```python
from build123d import *

# Parameters (mm, degrees)
BOSS_EXTRUDE1_DEPTH = 35.56
SKETCH2_W           = 2.54
SKETCH2_H           = 5.08
CUT_EXTRUDE1_DEPTH  = 10.16
SKETCH3_W           = 2.54
SKETCH3_H           = 5.08
CUT_EXTRUDE2_DEPTH  = 10.16
CHAMFER1_SIZE       = 0.508
FILLET1_R           = 0.635


with BuildPart() as part:
    # Sketch1 → Boss-Extrude1 (new body)
    with BuildSketch(Plane.XY):
        Polygon((-19.05, -0.3175), (-19.05, 0.3175), (-1.27, 0.3175), (-1.27, 5.3975), (1.27, 5.3975), (1.27, 0.3175), (19.05, 0.3175), (19.05, -0.3175), (1.27, -0.3175), (1.27, -0.635), (19.05, -0.635), (19.05, -1.27), (-19.05, -1.27), (-19.05, -0.635), (-1.27, -0.635), (-1.27, -0.3175), align=None)
    extrude(amount=-BOSS_EXTRUDE1_DEPTH)

    # Sketch2 → Cut-Extrude1 (cut)
    with BuildSketch(Plane.XY):
        with Locations((0, 2.8575)):
            Rectangle(SKETCH2_W, SKETCH2_H)
    extrude(amount=-CUT_EXTRUDE1_DEPTH, mode=Mode.SUBTRACT)

    # Sketch3 → Cut-Extrude2 (cut)
    with BuildSketch(Plane(origin=(0, 0, -35.56), x_dir=(-1, 0, 0), z_dir=(0, 0, -1))):
        with Locations((0, 2.8575)):
            Rectangle(SKETCH3_W, SKETCH3_H)
    extrude(amount=-CUT_EXTRUDE2_DEPTH, mode=Mode.SUBTRACT)

    # Chamfer1
    chamfer1_edges = [part.edges().sort_by_distance(p)[0] for p in [
        (0, 5.3975, -10.16),
        (1.27, 5.3975, -17.78),
        (-1.27, 5.3975, -17.78),
        (0, 5.3975, -25.4),
    ]]
    chamfer(chamfer1_edges, length=CHAMFER1_SIZE)

    # Fillet1
    fillet1_edges = [part.edges().sort_by_distance(p)[0] for p in [
        (1.27, 4.8895, -17.78),
        (0, 5.3975, -24.892),
        (-0.762, 5.3975, -17.78),
        (0, 5.3975, -10.668),
        (0.762, 5.3975, -17.78),
        (0, 4.8895, -10.16),
        (-1.27, 4.8895, -17.78),
        (0, 4.8895, -25.4),
    ]]
    fillet(fillet1_edges, radius=FILLET1_R)


solid = part.part
```
Check sheet for the modelled part. Datum: model origin and axes. Units: mm. A direction names the side the tool comes from. Coordinates: 2 decimals unless noted, no trailing zeros. Loops run counter-clockwise (first coordinate to the right, second up) from the corner with the lowest first, then second, coordinate; pieces in that order, holes last.
1) Material ranges on probe 1 along Y at (x, z) = (-12, -33.5) (1 decimal); probe 2 along X at (y, z) = (3.25, -22.5), recorded low to high.
2) Access from +Z, -Z, +X, -X, +Y, -Y to the whole of each face (thin tool, end or side, straight path). Record for faces 4 (the face through (0, 3, -10.16)), 5 (the face through (-1.27, 2, -18)), 6 (the face through (10, -0.318, -18)), 7 (the face through (-10, -0.318, -18)), 8 (the face through (0, 3, -25.4)).
3) Gauge pin test, flat ends, axial feed: pin 1 (1.5 mm diameter, centred on x = -8.5, z = -29, fed in from +Y); pin 2 (2 mm diameter, centred on x = 0, y = 2, fed in from -Z); pin 3 (1.3 mm diameter, centred on x = -0.5, y = 2.5, fed in from +Z). Record the tip position at first contact, or that the pin passes through.
4) Sectioned sample at C-C (y = 1.75). Record the boundary of the cut face in (x, z), and give its area (3 significant figures).
5) Sectioned sample at A-A (x = 2). Record the boundary of the cut face in (y, z) (1 decimal), and give its area (3 significant figures).
6) Release check for a two-part mould opening along Y. For faces 1 (the face through (10, -0.635, -18)), 2 (the face through (1.27, 3, -18)), 3 (the face through (0, 5.398, -18)) record: released by +Y, released by -Y, zero draft, split by the parting line, or undercut.
Check sheet entries:
1. probe 1: y = -1.3 to -0.6, -0.3 to 0.3
1. probe 2: x = -1.27 to 1.27
2. face 4: +Z, +X, -X, +Y
2. face 5: +Z, -Z, -X, +Y
2. face 6: +Z, -Z, +X
2. face 7: +Z, -Z, -X
2. face 8: -Z, +X, -X, +Y
3. pin 1: stops at y = 0.32
3. pin 2: stops at z = -25.4
3. pin 3: stops at z = -10.16
4. outline: (-1.27, -25.4) - (1.27, -25.4) - (1.27, -10.16) - (-1.27, -10.16) - close
4. area: 38.7 mm2
5. outline: (-1.3, -35.6) - (-0.6, -35.6) - (-0.6, 0) - (-1.3, 0) - close; (-0.3, -35.6) - (0.3, -35.6) - (0.3, 0) - (-0.3, 0) - close
5. area: 45.2 mm2
6. face 1: undercut
6. face 2: zero draft
6. face 3: released by +Y
